```python
from build123d import *

# Parameters (mm, degrees)
SKETCH1_R           = 10.25
BOSS_EXTRUDE1_DEPTH = 2
SKETCH2_R           = 4.5
SKETCH2_R_2         = 2.5
BOSS_EXTRUDE2_DEPTH = 3
SKETCH3_R           = 1.5
CUT_EXTRUDE1_DEPTH  = 16.333786225
SKETCH4_R           = 0.75
CUT_EXTRUDE2_DEPTH  = 16.333786225
CIRPATTERN1_COUNT   = 4


with BuildPart() as part:
    # Sketch1 → Boss-Extrude1 (new body)
    with BuildSketch(Plane(origin=(0, 0, 0), x_dir=(1, 0, 0), z_dir=(0, 1, 0))):
        with Locations(Location((0, 0, 0), (0, 0, 270))):
            Circle(SKETCH1_R)
    extrude(amount=BOSS_EXTRUDE1_DEPTH)

    # Sketch2 → Boss-Extrude2 (add)
    with BuildSketch(Plane(origin=(0, 2, 0), x_dir=(1, 0, 0), z_dir=(0, 1, 0))):
        with Locations(Location((0, 0, 0), (0, 0, 270))):
            Circle(SKETCH2_R)
        with Locations(Location((0, 0, 0), (0, 0, 270))):
            Circle(SKETCH2_R_2, mode=Mode.SUBTRACT)
    extrude(amount=BOSS_EXTRUDE2_DEPTH)

    # Sketch3 → Cut-Extrude1 (cut, through all)
    with BuildSketch(Plane.XZ):
        with Locations(Location((0, 0, 0), (0, 0, 270))):
            Circle(SKETCH3_R)
    extrude(amount=-CUT_EXTRUDE1_DEPTH, mode=Mode.SUBTRACT)

    # Sketch4 → Cut-Extrude2 (cut, through all)
    with BuildSketch(Plane.XZ):
        with Locations(Location((0, 7, 0), (0, 0, 270))):
            Circle(SKETCH4_R)
        with Locations(Location((-3.5, 7, 0), (0, 0, 270))):
            Circle(SKETCH4_R)
        with Locations(Location((3.5, 7, 0), (0, 0, 270))):
            Circle(SKETCH4_R)
    cut_extrude2 = extrude(amount=-CUT_EXTRUDE2_DEPTH, mode=Mode.SUBTRACT)

    # CirPattern1: Cut-Extrude2 ×4 about axis
    cirpattern1_axis = Axis((0, 0, 0), (0, 1, 0))
    for i in range(1, CIRPATTERN1_COUNT):
        add(cut_extrude2.rotate(cirpattern1_axis, i * 360 / CIRPATTERN1_COUNT), mode=Mode.SUBTRACT)


solid = part.part
```
The listing builds one solid part. Answer for the finished solid, in the listing's coordinates (mm). A direction names the side the tool comes from. Round coordinates to 2 decimals unless told otherwise and drop trailing zeros. Order: outer loops, then holes, each group sorted by start corner. A loop starts at its lowest first (then second) coordinate and runs counter-clockwise, first axis right, second up. Notation, with made-up numbers: (83, -20) -> (90, -20) arc R20 cw to (90, -14) -> close; hole circle Ø6 at (33, 52.25). An arc over 180 degrees is marked (long way). Answer as CSV lines item,"result". Start each with the question number.
(1) Find the intervals of material crossed by probe 1 along Z at (x, y) = (7, 1.15); probe 2 along X at (y, z) = (3.9, 0), in increasing order. Write a range as from..to.
(2) The part is cut by section A-A (x = 7). Determine the outline of the cut face in (y, z).
(3) The part is cut by section B-B (z = -0.5). Determine the outline of the cut face in (x, y).
(4) Flat-ended cylindrical pins translate along their axes: pin 1 Ø2 at (x, y) = (1.5, 0.5) entering from -Z; pin 2 Ø2 at (x, z) = (-3.5, -7) entering from +Y; pin 3 Ø1.2 at (x, z) = (-3.5, 7) entering from -Y; pin 4 Ø1 at (x, y) = (-2, 2) entering from +Z. Find the tip coordinate at first contact, or state that the pin passes through.
(5) The part is cut by section C-C (x = 3.5). Determine the outline of the cut face in (y, z).
(6) A tool of negligible diameter and unlimited length cuts with its end or side. For faces 1 (the face through (-2.44, 3.48, -0.54)), 2 (the face through (-3.956, 0.986, 7.595)), from which of +Z, -Z, +X, -X, +Y, -Y can it reach the whole face along a straight path? Write none if from no direction.
(7) For a pull along Z with two mould halves and no side action, classify faces 3 (the face through (3.044, 0.986, 7.595)), 4 (the face through (1.352, 3.479, 4.292)), 5 (the face through (-2, 5, 2)) as +Z half, -Z half, draft (parallel to the pull), parting line (faces both ways), or undercut.
(8) The part is cut by section D-D (z = 3.5). Determine the outline of the cut face in (x, y), then the cut area to 3 significant figures.
Evaluation:
1,probe 1,"-7.49..-4.25, -2.75..-0.75, 0.75..2.75, 4.25..7.49"
1,probe 2,"-4.5..-2.5, 2.5..4.5"
2,outline,"(0, -7.49) -> (2, -7.49) -> (2, -4.25) -> (0, -4.25) -> close; (0, -2.75) -> (2, -2.75) -> (2, -0.75) -> (0, -0.75) -> close; (0, 0.75) -> (2, 0.75) -> (2, 2.75) -> (0, 2.75) -> close; (0, 4.25) -> (2, 4.25) -> (2, 7.49) -> (0, 7.49) -> close"
3,outline,"(-10.24, 0) -> (-7.56, 0) -> (-7.56, 2) -> (-10.24, 2) -> close; (-6.44, 0) -> (-1.41, 0) -> (-1.41, 2) -> (-2.45, 2) -> (-2.45, 5) -> (-4.47, 5) -> (-4.47, 2) -> (-6.44, 2) -> close; (1.41, 0) -> (6.44, 0) -> (6.44, 2) -> (4.47, 2) -> (4.47, 5) -> (2.45, 5) -> (2.45, 2) -> (1.41, 2) -> close; (7.56, 0) -> (10.24, 0) -> (10.24, 2) -> (7.56, 2) -> close"
4,pin 1,"z = -10.24"
4,pin 2,"y = 2"
4,pin 3,"through"
4,pin 4,"z = 10.14"
5,outline,"(0, -9.63) -> (2, -9.63) -> (2, -7.75) -> (0, -7.75) -> close; (0, -6.25) -> (2, -6.25) -> (2, -2.83) -> (5, -2.83) -> (5, 2.83) -> (2, 2.83) -> (2, 6.25) -> (0, 6.25) -> close; (0, 7.75) -> (2, 7.75) -> (2, 9.63) -> (0, 9.63) -> close"
6,face 1,"+Y"
6,face 2,"+Y, -Y"
7,face 3,"undercut"
7,face 4,"parting line"
7,face 5,"draft"
8,outline,"(-9.63, 0) -> (-7.75, 0) -> (-7.75, 2) -> (-9.63, 2) -> close; (-6.25, 0) -> (6.25, 0) -> (6.25, 2) -> (2.83, 2) -> (2.83, 5) -> (-2.83, 5) -> (-2.83, 2) -> (-6.25, 2) -> close; (7.75, 0) -> (9.63, 0) -> (9.63, 2) -> (7.75, 2) -> close"
8,area,"49.5 mm²"
